Autodesk Inventor part; units mm, degrees
ref_plane "РабПлоскость1" through (0, 0, 175) normal (0, 0, -1) x (-1, 0, 0)
ref_plane "РабПлоскость2" through (0, 0, 175) normal (0, 0, -1) x (-1, 0, 0)
ref_plane "YZ Plane" through (0, 0, 0) normal (1, 0, 0) x (0, 1, 0)
sketch "Эскиз1" plane through (0, 0, 0) normal (0, 0, 1) x (1, 0, 0)
  circle A0 centre (0, 0) radius 175
  line L0 (0, 136) -> (87.5, 136)
  line L1 (87.5, 136) -> (-87.5, 136)
  line L2 (-87.5, 151.5544) -> (-87.5, 142)
  line L3 (-87.5, 142) -> (87.5, 142)
  line L4 (87.5, 142) -> (87.5, 151.5544)
  dimension "d0" = 350
  dimension "d1" = 87.5
  dimension "d2" = 175
  dimension "d13" = 142
extrude "Выдавливание1" add sketch "Эскиз1" along normal blind 350 contours L4 L3 L2 A0 picked at (0, 153)
ref_plane "РабПлоскость1" through (0, 0, 175) normal (0, 0, -1) x (-1, 0, 0)
sketch "Эскиз2" plane through (0, 0, 175) normal (0, 0, -1) x (-1, 0, 0)
  arc A0 (87.5, 151.5544) -> (-87.5, 151.5544) centre (0, 0) ccw
  line L0 (-87.5, 142) -> (-87.5, 151.5544)
  arc A1 (87.5, 151.5544) -> (-87.5, 151.5544) centre (0, 0) ccw
  line L1 (87.5, 151.5544) -> (87.5, 142)
  line L2 (87.5, 142) -> (-87.5, 142)
  circle A2 centre (0, 0) radius 162.5
  line L3 (87.5, 142) -> (-87.5, 142)
  line L4 (0, 142) -> (-6, 142)
  line L5 (-6, 142) -> (-6, 162.3892)
  line L6 (0, 142) -> (6, 142)
  line L7 (6, 142) -> (6, 162.3892)
  point P0 (-79.0079, 142)
  point P1 (79.0079, 142)
  dimension "d7" = 325
  dimension "d8" = 6
  dimension "d9" = 6
extrude "Выдавливание2" cut sketch "Эскиз2" against normal mid plane 320 contours L2 L7 A2 | A2 L5 L2
fillet "Сопряжение1" radius 5 10 edges at (-43.7095, 156.5111, 335) (43.7095, 156.5111, 335) (-6, 162.3892, 175) (-6, 152.1946, 335) (6, 162.3892, 175) (6, 152.1946, 335) (6, 152.1946, 15) (43.7095, 156.5111, 15) (-43.7095, 156.5111, 15) (-6, 152.1946, 15)
sketch "Эскиз3" plane through (-87.5, 142, 0) normal (0, -1, 0) x (1, 0, 0)
  line L0 (175, 0) -> (175, 8)
  line L1 (175, 0) -> (175, 350)
  line L2 (175, 8) -> (167, 8)
  dimension "d14" = 8
hole "Отверстие1" at (79.5, 142, 8) direction (0, 1, 0) diameter 5 depth 8 tip angle 118 counterbore diameter 6 counterbore depth 6
mirror "Зеркальное отражение1" about plane through (0, 0, 0) normal (1, 0, 0) of "Отверстие1"
ref_plane "РабПлоскость2" through (0, 0, 175) normal (0, 0, -1) x (-1, 0, 0)
mirror "Зеркальное отражение2" about plane through (0, 0, 175) normal (0, 0, -1) of "Отверстие1", "Зеркальное отражение1"
thread "Резьба1"
thread "Резьба2"
thread "Резьба3"
thread "Резьба4"
properties part number "Башмак_CPY" material "Бронза, мягкое олово"
Work out the finished part from the listing and answer in its coordinate system (mm). A direction names the side the tool comes from. Give positions to 0.01 mm unless a question says otherwise; leave off trailing zeros. Order: outer loops, then holes, each group sorted by start corner. A loop starts at its lowest first (then second) coordinate and runs counter-clockwise, first axis right, second up. Notation, with made-up numbers: (41, 78.25) -> (56, 78.25) arc R26 cw to (56, 112.25) -> close; hole circle Ø9 at (30, 75). An arc over 180 degrees is marked (long way). Answer as a JSON object with one key per item and string values. Group by question number.
1. A tool of negligible diameter and unlimited length cuts with its end or side. For faces 4 (the cylindrical face through (-1.283, 174.995, 172.55)), 5 (the flat face through (-77, 148, 7)), from which of +Z, -Z, +X, -X, +Y, -Y can it reach the whole face along a straight path? Write none if from no direction.
2. Consider line 1 along Z through (x, y) = (79.5, 148.7); line 2 along X through (y, z) = (146, 342); line 3 along Z through (x, y) = (79.5, 144.5). Determine where each line is inside the solid, lowest interval first. Write a range as [from, to].
3. The mould has two halves that part along Z. Classify faces 1 (the flat face through (-33, 148, 335)), 2 (the flat face through (-1, 155, 0)), 3 (the flat face through (-1, 155, 350)): released by +Z, released by -Z, zero draft, split by the parting line, or undercut.
4. Flat-ended cylindrical pins translate along their axes: pin 1 Ø5.5 at (x, z) = (79.5, 342) entering from +Y; pin 2 Ø4 at (y, z) = (154, 188.5) entering from +X; pin 3 Ø1.5 at (x, z) = (-38.5, 210) entering from -Y. Find the tip coordinate at first contact, or state that the pin passes through.
5. Section A-A on z = 190 is taken. Determine the outline of the cut face in (x, y), plus the area to 3 significant figures.
Result sheet:
{
 "1": {"face 4": "+Z, -Z, +Y", "face 5": "-Y"},
 "2": {"line 1": "z = [0, 5.5], [10.5, 339.5], [344.5, 350]", "line 2": "x = [-87.5, -82.5], [-76.5, 76.5], [82.5, 87.5]", "line 3": "z = [0, 5], [11, 339], [345, 350]"},
 "3": {"face 1": "undercut", "face 2": "released by -Z", "face 3": "released by +Z"},
 "4": {"pin 1": "stops at y = 157.27", "pin 2": "stops at x = 86.72", "pin 3": "stops at y = 157.69"},
 "5": {"outline": "(-87.5, 142) -> (-79.01, 142) arc R162.5 cw to (-11.35, 162.1) arc R5 cw to (-6, 157.12) -> (-6, 142) -> (6, 142) -> (6, 157.12) arc R5 cw to (11.35, 162.1) arc R162.5 cw to (79.01, 142) -> (87.5, 142) -> (87.5, 151.55) arc R175 ccw to (-87.5, 151.55) -> close", "area": "2,520 mm^2"}
}
